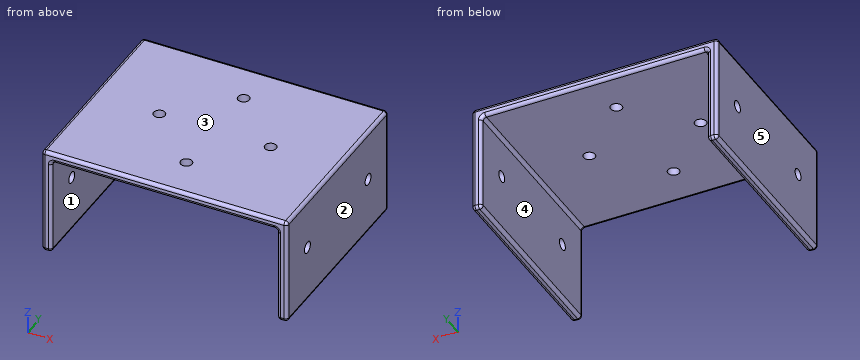
```python
from build123d import *

# Parameters (mm, degrees)
SKETCH1_W           = 75
SKETCH1_H           = 60
BOSS_EXTRUDE1_DEPTH = 3
SKETCH2_W           = 3
SKETCH2_H           = 60
BOSS_EXTRUDE2_DEPTH = 30
SKETCH3_R           = 1.75
CUT_EXTRUDE1_DEPTH  = 30
FILLET1_R           = 1
SKETCH4_R           = 1.75
CUT_EXTRUDE2_DEPTH  = 87.168439698


with BuildPart() as part:
    # Sketch1 → Boss-Extrude1 (new body)
    with BuildSketch(Plane.XY):
        Rectangle(SKETCH1_W, SKETCH1_H)
    extrude(amount=BOSS_EXTRUDE1_DEPTH)

    # Sketch2 → Boss-Extrude2 (add)
    with BuildSketch(Plane(origin=(0, 0, 0), x_dir=(-1, 0, 0), z_dir=(0, 0, -1))):
        with Locations((-36, 0)):
            Rectangle(SKETCH2_W, SKETCH2_H)
    boss_extrude2 = extrude(amount=BOSS_EXTRUDE2_DEPTH)

    # Mirror1: Boss-Extrude2 across plane
    add(boss_extrude2.mirror(Plane(origin=(0, 0, 0), x_dir=(0, 0, 1), z_dir=(1, 0, 0))))

    # Sketch3 → Cut-Extrude1 (cut)
    with BuildSketch(Plane.XY.offset(3)):
        with Locations((0, 17)):
            Circle(SKETCH3_R)
        with Locations((17, 0)):
            Circle(SKETCH3_R)
        with Locations((0, -17)):
            Circle(SKETCH3_R)
        with Locations((-17, 0)):
            Circle(SKETCH3_R)
    extrude(amount=-CUT_EXTRUDE1_DEPTH, mode=Mode.SUBTRACT)

    # Fillet1
    fillet1_edges = [part.edges().sort_by_distance(p)[0] for p in [
        (-37.5, 0, 3),
        (0, 30, 0),
        (34.5, 0, 0),
        (34.5, -30, -15),
        (34.5, 30, -15),
        (37.5, 0, -30),
        (0, -30, 3),
        (36, -30, -30),
        (34.5, 0, -30),
        (36, 30, -30),
        (0, -30, 0),
        (-37.5, 0, -30),
        (-36, 30, -30),
        (-34.5, 0, -30),
        (-34.5, 30, -15),
        (-36, -30, -30),
        (-34.5, -30, -15),
        (-34.5, 0, 0),
        (37.5, 0, 3),
        (37.5, -30, -13.5),
        (-37.5, -30, -13.5),
        (-37.5, 30, -13.5),
        (37.5, 30, -13.5),
        (0, 30, 3),
    ]]
    fillet(fillet1_edges, radius=FILLET1_R)

    # Sketch4 → Cut-Extrude2 (cut, through all)
    with BuildSketch(Plane(origin=(37.5, 0, 0), x_dir=(0, 0, -1), z_dir=(1, 0, 0))):
        with Locations((12.5, 18)):
            Circle(SKETCH4_R)
        with Locations((12.5, -18)):
            Circle(SKETCH4_R)
    extrude(amount=-CUT_EXTRUDE2_DEPTH, mode=Mode.SUBTRACT)


solid = part.part
```
Source: CAD feature listing. Evaluate the final solid. Frame: model axes, mm. Face numbers are marked on the shaded views. A direction names the side the tool comes from. Coordinates: 2 decimals unless noted, no trailing zeros. Write each loop counter-clockwise with the first axis right and the second up, starting at its lowest first coordinate (ties: lowest second). Pieces come first, ordered by that corner, then holes. Notation, with made-up numbers: (24.5, -17) -> (37.5, -17) arc R19 cw to (37.5, 17) -> close; hole circle Ø2 at (-37, 0). An arc over 180 degrees is marked (long way). Return JSON: item names as keys, results as strings. Group by question number.
1) Section query B-B, the plane z = -12.5. State how many separate pieces and enclosed holes the cut face has, plus the area to 3 significant figures.
2) Contact query for flat-ended pins moving along their axis: P1, Ø8, axis at x = -17, z = -2, coming from the +Y side; P2, Ø17.5, axis at x = -8.5, y = -9, coming from the -Z side. Output: stop coordinate, or through.
3) Section query D-D, the plane z = -6. Return loops of the section in (x, y).
4) Mould query, pull axis X, two halves, no side actions, for the marked faces 1, 2 and 3. Classes: +X half, -X half, draft (parallel to the pull), parting line (faces both ways), or undercut.
5) Ray query, line 1 along Y through (x, z) = (36, -12.5); line 2 along X through (y, z) = (-10, -16); line 3 along Y through (x, z) = (-35, -12). Return the intervals inside material, ascending.
6) Section query C-C, the plane x = 0. Return loops of the section in (y, z).
7) Section query A-A, the plane x = 17. Return loops of the section in (y, z).
8) Set-up query: the marked faces 4 and 5. Return all of +Z, -Z, +X, -X, +Y, -Y with unobstructed straight access to the full face (end or side cutting, diameter ignored); none if empty.
From the geometry:
{
 "1": {"separate pieces": "6", "enclosed holes": "0", "area": "316 mm²"},
 "2": {"P1": "y = 30", "P2": "z = 0"},
 "3": {"outline": "(-37.5, -29) arc R1 ccw to (-36.5, -30) -> (-35.5, -30) arc R1 ccw to (-34.5, -29) -> (-34.5, 29) arc R1 ccw to (-35.5, 30) -> (-36.5, 30) arc R1 ccw to (-37.5, 29) -> close; (34.5, -29) arc R1 ccw to (35.5, -30) -> (36.5, -30) arc R1 ccw to (37.5, -29) -> (37.5, 29) arc R1 ccw to (36.5, 30) -> (35.5, 30) arc R1 ccw to (34.5, 29) -> close"},
 "4": {"face 1": "undercut", "face 2": "+X half", "face 3": "draft"},
 "5": {"line 1": "-30 to -19.75, -16.25 to 16.25, 19.75 to 30", "line 2": "-37.5 to -34.5, 34.5 to 37.5", "line 3": "-29.87 to -19.68, -16.32 to 16.32, 19.68 to 29.87"},
 "6": {"outline": "(-30, 1) arc R1 ccw to (-29, 0) -> (-18.75, 0) -> (-18.75, 3) -> (-29, 3) arc R1 ccw to (-30, 2) -> close; (-15.25, 0) -> (15.25, 0) -> (15.25, 3) -> (-15.25, 3) -> close; (18.75, 0) -> (29, 0) arc R1 ccw to (30, 1) -> (30, 2) arc R1 ccw to (29, 3) -> (18.75, 3) -> close"},
 "7": {"outline": "(-30, 1) arc R1 ccw to (-29, 0) -> (-1.75, 0) -> (-1.75, 3) -> (-29, 3) arc R1 ccw to (-30, 2) -> close; (1.75, 0) -> (29, 0) arc R1 ccw to (30, 1) -> (30, 2) arc R1 ccw to (29, 3) -> (1.75, 3) -> close"},
 "8": {"face 4": "-Z, +Y, -Y", "face 5": "+Z, -Z, -X, +Y, -Y"}
}
